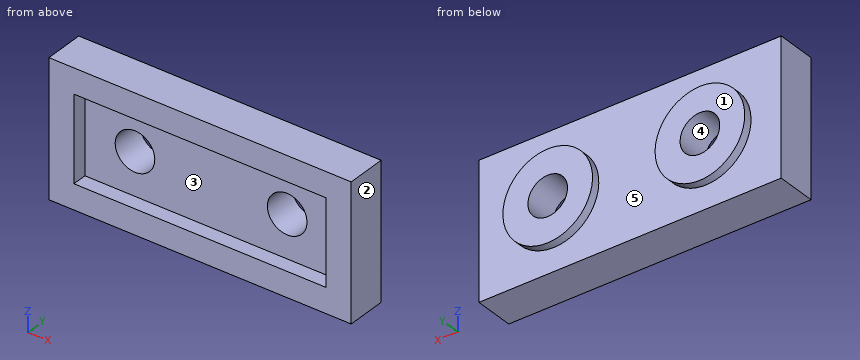
from build123d import *

# Parameters (mm, degrees)
SKETCH1_W           = 14.5
SKETCH1_H           = 6.5
BOSS_EXTRUDE1_DEPTH = 1.9
SHELL1_T            = -1.2
SKETCH2_R           = 2.15
SKETCH2_R_2         = 0.95
BOSS_EXTRUDE2_DEPTH = 0.4
CUT_EXTRUDE1_START  = -3.4
SKETCH3_R           = 0.95
CUT_EXTRUDE1_DEPTH  = 3.4
CUT_EXTRUDE2_START  = -3.4
SKETCH4_R           = 0.95
CUT_EXTRUDE2_DEPTH  = 3.4


with BuildPart() as part:
    # Sketch1 → Boss-Extrude1 (new body)
    with BuildSketch(Plane(origin=(0, 0, 0), x_dir=(1, 0, 0), z_dir=(0, 1, 0))):
        Rectangle(SKETCH1_W, SKETCH1_H)
    extrude(amount=BOSS_EXTRUDE1_DEPTH)

    # Shell1
    shell1_openings = [part.faces().sort_by_distance(p)[0] for p in [
        (0, 0, 0),
    ]]
    offset(amount=SHELL1_T, openings=shell1_openings, kind=Kind.INTERSECTION)

    # Sketch2 → Boss-Extrude2 (add)
    # profile 1 of 2: a face of its own
    with BuildSketch(Plane(origin=(0, 1.9, 0), x_dir=(1, 0, 0), z_dir=(0, 1, 0))):
        with Locations(Location((-3.65, 0, 0), (0, 0, 270))):
            Circle(SKETCH2_R)
        with Locations(Location((-3.65, 0, 0), (0, 0, 270))):
            Circle(SKETCH2_R_2, mode=Mode.SUBTRACT)
    # profile 2 of 2: a face of its own
    with BuildSketch(Plane(origin=(0, 1.9, 0), x_dir=(1, 0, 0), z_dir=(0, 1, 0))):
        with Locations(Location((3.65, 0, 0), (0, 0, 90))):
            Circle(SKETCH2_R)
        with Locations(Location((3.65, 0, 0), (0, 0, 90))):
            Circle(SKETCH2_R_2, mode=Mode.SUBTRACT)
    extrude(amount=BOSS_EXTRUDE2_DEPTH)

    # Sketch3 → Cut-Extrude1 (cut)
    with BuildSketch(Plane(origin=(0, 1.9, 0), x_dir=(1, 0, 0), z_dir=(0, 1, 0)).offset(CUT_EXTRUDE1_START)):
        with Locations(Location((-3.65, 0, 0), (0, 0, 270))):
            Circle(SKETCH3_R)
    extrude(amount=CUT_EXTRUDE1_DEPTH, mode=Mode.SUBTRACT)

    # Sketch4 → Cut-Extrude2 (cut)
    with BuildSketch(Plane(origin=(0, 1.9, 0), x_dir=(1, 0, 0), z_dir=(0, 1, 0)).offset(CUT_EXTRUDE2_START)):
        with Locations(Location((3.65, 0, 0), (0, 0, 90))):
            Circle(SKETCH4_R)
    extrude(amount=CUT_EXTRUDE2_DEPTH, mode=Mode.SUBTRACT)


solid = part.part
The model under review builds one solid part; all positions refer to its coordinate system, in mm. Face numbers are marked on the shaded views. A direction names the side the tool comes from. Give positions to 0.01 mm unless a question says otherwise; leave off trailing zeros. Order: outer loops, then holes, each group sorted by start corner. A loop starts at its lowest first (then second) coordinate and runs counter-clockwise, first axis right, second up. Notation, with made-up numbers: M -28,-19 L 18,-19 A32 ccw 18,13 Z; hole C 89.25,14 d4. An arc over 180 degrees is marked long. Answer in a Markdown table with one row per item. Add a question column.
1. To check wall thickness, follow line 1 along X through (y, z) = (1, 0); line 2 along Z through (x, y) = (-3.65, 1.6); line 3 along X through (y, z) = (0.6, 1.25). State the ranges of each line that lie inside material, in increasing order.
2. Add section C-C on x = -0.5. State the section outline as (y, z) points, plus the area to 3 significant figures.
3. For pin 1 Ø2.5 at (x, z) = (3.65, 0) entering from -Y, flat-tipped, find the tip position at first contact; note if it passes through.
4. Add section A-A on x = -3.65. State the section outline as (y, z) points.
5. Add section B-B on z = 0. State the section outline as (x, y) points.
6. Machinability: for the marked faces 4 and 5, which of the approach directions +Z, -Z, +X, -X, +Y, -Y give a long, thin tool a straight path to every point of the face, cutting with its end or side? Answer none if there is none.
7. Mouldability with a two-part tool opening along X and no side actions: class the marked faces 1, 2 and 3 as released by +X, released by -X, zero draft, split by the parting line, or undercut.
8. Add section D-D on y = 1.75. State the section outline as (x, z) points.
The answers:
| question | item | result |
|---|---|---|
| 1 | line 1 | -7.25 to -4.6, -2.7 to 2.7, 4.6 to 7.25 |
| 1 | line 2 | -3.25 to -0.95, 0.95 to 3.25 |
| 1 | line 3 | -7.25 to -6.05, 6.05 to 7.25 |
| 2 | outline | M 0,-3.25 L 1.9,-3.25 L 1.9,3.25 L 0,3.25 L 0,2.05 L 0.7,2.05 L 0.7,-2.05 L 0,-2.05 Z |
| 2 | area | 9.48 mm2 |
| 3 | pin 1 | y = 0.7 |
| 4 | outline | M 0,-3.25 L 1.9,-3.25 L 1.9,-2.15 L 2.3,-2.15 L 2.3,-0.95 L 0.7,-0.95 L 0.7,-2.05 L 0,-2.05 Z; M 0,2.05 L 0.7,2.05 L 0.7,0.95 L 2.3,0.95 L 2.3,2.15 L 1.9,2.15 L 1.9,3.25 L 0,3.25 Z |
| 5 | outline | M -7.25,0 L -6.05,0 L -6.05,0.7 L -4.6,0.7 L -4.6,2.3 L -5.8,2.3 L -5.8,1.9 L -7.25,1.9 Z; M -2.7,0.7 L 2.7,0.7 L 2.7,2.3 L 1.5,2.3 L 1.5,1.9 L -1.5,1.9 L -1.5,2.3 L -2.7,2.3 Z; M 4.6,0.7 L 6.05,0.7 L 6.05,0 L 7.25,0 L 7.25,1.9 L 5.8,1.9 L 5.8,2.3 L 4.6,2.3 Z |
| 6 | face 4 | +Y, -Y |
| 6 | face 5 | +Y |
| 7 | face 1 | zero draft |
| 7 | face 2 | released by +X |
| 7 | face 3 | undercut |
| 8 | outline | M -7.25,-3.25 L 7.25,-3.25 L 7.25,3.25 L -7.25,3.25 Z; hole C -3.65,0 d1.9; hole C 3.65,0 d1.9 |
